Part model, mm, in its own coordinate system. Round coordinates to 2 decimals unless told otherwise and drop trailing zeros. Write each loop counter-clockwise with the first axis right and the second up, starting at its lowest first coordinate (ties: lowest second). Pieces come first, ordered by that corner, then holes. Notation, with made-up numbers: M 80,32 L 116,32 A20 cw 116,52 Z; hole C 83,-21 d4. An arc over 180 degrees is marked long. One line per question, with ' | ' between items. Start each with the question number.
1) Saw through at B-B (y = 0). List the corners of the cut face in (x, z), plus the area to 3 significant figures.
2) Saw through at D-D (y = -9). List the corners of the cut face in (x, z).
3) Saw through at C-C (z = -1.15). List the corners of the cut face in (x, y).
4) Saw through at A-A (x = 0). List the corners of the cut face in (y, z), plus the area to 3 significant figures.
5) Wall check: probe 1 along X at (y, z) = (0, -0.7); probe 2 along Y at (x, z) = (0, -1.85); probe 3 along X at (y, z) = (12, -1). Give the ranges that are in metal, low to high. Write a range as [from, to].
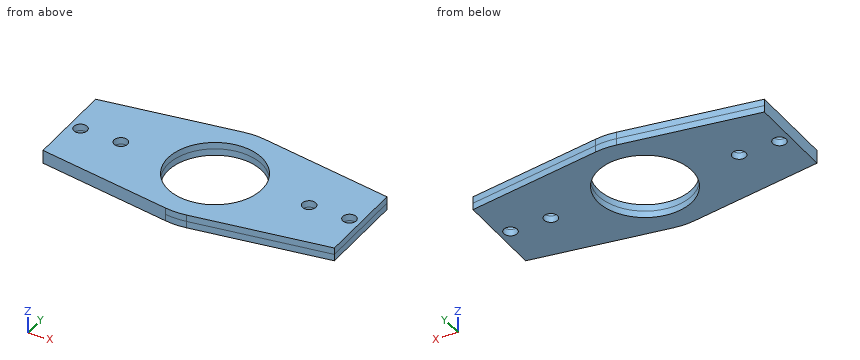
```python
from build123d import *
from build123d.topology import SkipClean

# Parameters (mm, degrees)
SKETCH1_R           = 3.000000000000015
SKETCH1_R_2         = 3.0000000000000013
SKETCH1_R_3         = 3.0000000000000084
SKETCH1_R_4         = 16
BOSS_EXTRUDE1_DEPTH = 6
BOSS_EXTRUDE3_START = 3.5
SKETCH3_R           = 30.000000000000057
SKETCH3_R_2         = 21
BOSS_EXTRUDE3_DEPTH = 3.5
BOSS_EXTRUDE4_START = 3.5
SKETCH4_R           = 3.000000000000015
SKETCH4_R_2         = 3.0000000000000013
SKETCH4_R_3         = 3.0000000000000084
BOSS_EXTRUDE4_DEPTH = 3.5
SKETCH5_R           = 3.000000000000015
SKETCH5_R_2         = 3.0000000000000013
SKETCH5_R_3         = 21
SKETCH5_R_4         = 3.0000000000000084
CUT_EXTRUDE1_DEPTH  = 0.5
CUT_EXTRUDE2_DEPTH  = 182.00000000000009
SKETCH7_R           = 21
CUT_EXTRUDE3_DEPTH  = 10


with BuildPart() as part:
    # Sketch1 → Boss-Extrude1 (new body)
    with BuildSketch(Plane.XY):
        with BuildLine():
            Line((-65.00000000000001, 20), (-65, -20))
            Line((-65, -20), (-4.73088284384841, -29.624630757492685))
            ThreePointArc((-4.73088284384841, -29.624630757492685), (1.516e-14, -30.000000000000014), (4.7308828438484465, -29.624630757492678))
            Line((4.7308828438484465, -29.624630757492678), (65.00000000000003, -19.99999999999992))
            Line((65.00000000000003, -19.99999999999992), (65.00000000000001, 20))
            Line((65.00000000000001, 20), (4.730882843848428, 29.624630757492728))
            ThreePointArc((4.730882843848428, 29.624630757492728), (1.84e-15, 30.00000000000006), (-4.730882843848428, 29.624630757492728))
            Line((-4.730882843848428, 29.624630757492728), (-65.00000000000001, 20))
        make_face()
        with Locations((59.99999999998411, -4.545e-13)):
            Circle(SKETCH1_R, mode=Mode.SUBTRACT)
        with Locations((42, 0)):
            Circle(SKETCH1_R_2, mode=Mode.SUBTRACT)
        with Locations(Location((-59.99999999998411, -4.545e-13, 0), (0, 0, 180))):
            Circle(SKETCH1_R_3, mode=Mode.SUBTRACT)
        with Locations(Location((-42, 0, 0), (0, 0, 180))):
            Circle(SKETCH1_R_2, mode=Mode.SUBTRACT)
        Circle(SKETCH1_R_4, mode=Mode.SUBTRACT)
    extrude(amount=BOSS_EXTRUDE1_DEPTH)

    # Sketch3 → Boss-Extrude3 (add)
    with SkipClean():  # the faces are left unmerged after this step: merging them gives an invalid solid
        with BuildSketch(Plane(origin=(0, 0, 0), x_dir=(-1, 0, 0), z_dir=(0, 0, -1)).offset(BOSS_EXTRUDE3_START)):
            Circle(SKETCH3_R)
            Circle(SKETCH3_R_2, mode=Mode.SUBTRACT)
        extrude(amount=-BOSS_EXTRUDE3_DEPTH)

    # Sketch4 → Boss-Extrude4 (add)
    # profile 1 of 2: a face of its own
    with BuildSketch(Plane(origin=(0, 0, 0), x_dir=(-1, 0, 0), z_dir=(0, 0, -1)).offset(BOSS_EXTRUDE4_START)):
        with BuildLine():
            Line((4.730882843848405, -29.624630757492703), (65, -20))
            Line((65, -20), (65.00000000000001, 20))
            Line((65.00000000000001, 20), (4.730882843848438, 29.624630757492703))
            ThreePointArc((4.730882843848438, 29.624630757492703), (30.000000000000032, -1.998e-14), (4.730882843848405, -29.624630757492703))
        make_face()
        with Locations((59.99999999998411, -4.545e-13)):
            Circle(SKETCH4_R, mode=Mode.SUBTRACT)
        with Locations((42, 0)):
            Circle(SKETCH4_R_2, mode=Mode.SUBTRACT)
    # profile 2 of 2: a face of its own
    with BuildSketch(Plane(origin=(0, 0, 0), x_dir=(-1, 0, 0), z_dir=(0, 0, -1)).offset(BOSS_EXTRUDE4_START)):
        with BuildLine():
            Line((-4.730882843848428, 29.624630757492703), (-65.00000000000001, 20))
            Line((-65.00000000000001, 20), (-65.00000000000003, -19.99999999999992))
            Line((-65.00000000000003, -19.99999999999992), (-4.730882843848441, -29.624630757492703))
            ThreePointArc((-4.730882843848441, -29.624630757492703), (-30.000000000000036, 3.67e-15), (-4.730882843848428, 29.624630757492703))
        make_face()
        with Locations((-42, 0)):
            Circle(SKETCH4_R_2, mode=Mode.SUBTRACT)
        with Locations((-59.99999999998411, -4.545e-13)):
            Circle(SKETCH4_R_3, mode=Mode.SUBTRACT)
    extrude(amount=-BOSS_EXTRUDE4_DEPTH)

    # Sketch5 → Cut-Extrude1 (cut)
    with BuildSketch(Plane(origin=(0, 0, -3.5), x_dir=(-1, 0, 0), z_dir=(0, 0, -1))):
        with BuildLine():
            Line((-4.730882843848428, 29.624630757492703), (-65.00000000000001, 20))
            Line((-65.00000000000001, 20), (-65.00000000000003, -19.99999999999992))
            Line((-65.00000000000003, -19.99999999999992), (-4.73088284384847, -29.6246307574927))
            ThreePointArc((-4.73088284384847, -29.6246307574927), (-3.147e-14, -30.00000000000004), (4.730882843848405, -29.624630757492703))
            Line((4.730882843848405, -29.624630757492703), (65, -20))
            Line((65, -20), (65.00000000000001, 20))
            Line((65.00000000000001, 20), (4.730882843848431, 29.624630757492703))
            ThreePointArc((4.730882843848431, 29.624630757492703), (1.84e-15, 30.000000000000036), (-4.730882843848428, 29.624630757492703))
        make_face()
        with Locations((59.99999999998411, -4.545e-13)):
            Circle(SKETCH5_R, mode=Mode.SUBTRACT)
        with Locations((42, 0)):
            Circle(SKETCH5_R_2, mode=Mode.SUBTRACT)
        Circle(SKETCH5_R_3, mode=Mode.SUBTRACT)
        with Locations((-42, 0)):
            Circle(SKETCH5_R_2, mode=Mode.SUBTRACT)
        with Locations((-59.99999999998411, -4.545e-13)):
            Circle(SKETCH5_R_4, mode=Mode.SUBTRACT)
    extrude(amount=-CUT_EXTRUDE1_DEPTH, mode=Mode.SUBTRACT)

    # Sketch6 → Cut-Extrude2 (cut)
    with BuildSketch(Plane(origin=(65.00000000000003, 2.255e-14, 0), x_dir=(0, 0, -1), z_dir=(1, 3.5e-16, 0))):
        Polygon((-3, 36.68379412989912), (-2.999999999999992, -32.31620587010089), (-5.999999999999992, -32.31620587010089), (-6, 29.812315378746394), (-6, 36.68379412989912), align=None)
    extrude(amount=-CUT_EXTRUDE2_DEPTH, mode=Mode.SUBTRACT)

    # Sketch7 → Cut-Extrude3 (cut)
    with BuildSketch(Plane(origin=(0, 0, 0), x_dir=(-1, 0, 0), z_dir=(0, 0, -1))):
        with Locations(Location((0, 0, 0), (0, 0, 90))):
            Circle(SKETCH7_R)
    extrude(amount=-CUT_EXTRUDE3_DEPTH, mode=Mode.SUBTRACT)


solid = part.part
```
Answer key:
1) outline: M -65,-3 L -63,-3 L -63,3 L -65,3 Z; M -57,-3 L -45,-3 L -45,3 L -57,3 Z; M -39,-3 L -21,-3 L -21,3 L -39,3 Z; M 21,-3 L 39,-3 L 39,3 L 21,3 Z; M 45,-3 L 57,-3 L 57,3 L 45,3 Z; M 63,-3 L 65,-3 L 65,3 L 63,3 Z | area: 384 mm2
2) outline: M -65,-3 L -18.97,-3 L -18.97,3 L -65,3 Z; M 18.97,-3 L 65,-3 L 65,3 L 18.97,3 Z
3) outline: M -65,-20 L -4.73,-29.62 A30 ccw 4.73,-29.62 L 65,-20 L 65,20 L 4.73,29.62 A30 ccw -4.73,29.62 L -65,20 Z; hole C -60,0 d6; hole C -42,0 d6; hole C 0,0 d42; hole C 42,0 d6; hole C 60,0 d6
4) outline: M -30,-3 L -21,-3 L -21,3 L -30,3 Z; M 21,-3 L 30,-3 L 30,3 L 21,3 Z | area: 108 mm2
5) probe 1: x = [-65, -63], [-57, -45], [-39, -21], [21, 39], [45, 57], [63, 65] | probe 2: y = [-30, -21], [21, 30] | probe 3: x = [-65, -17.23], [17.23, 65]
